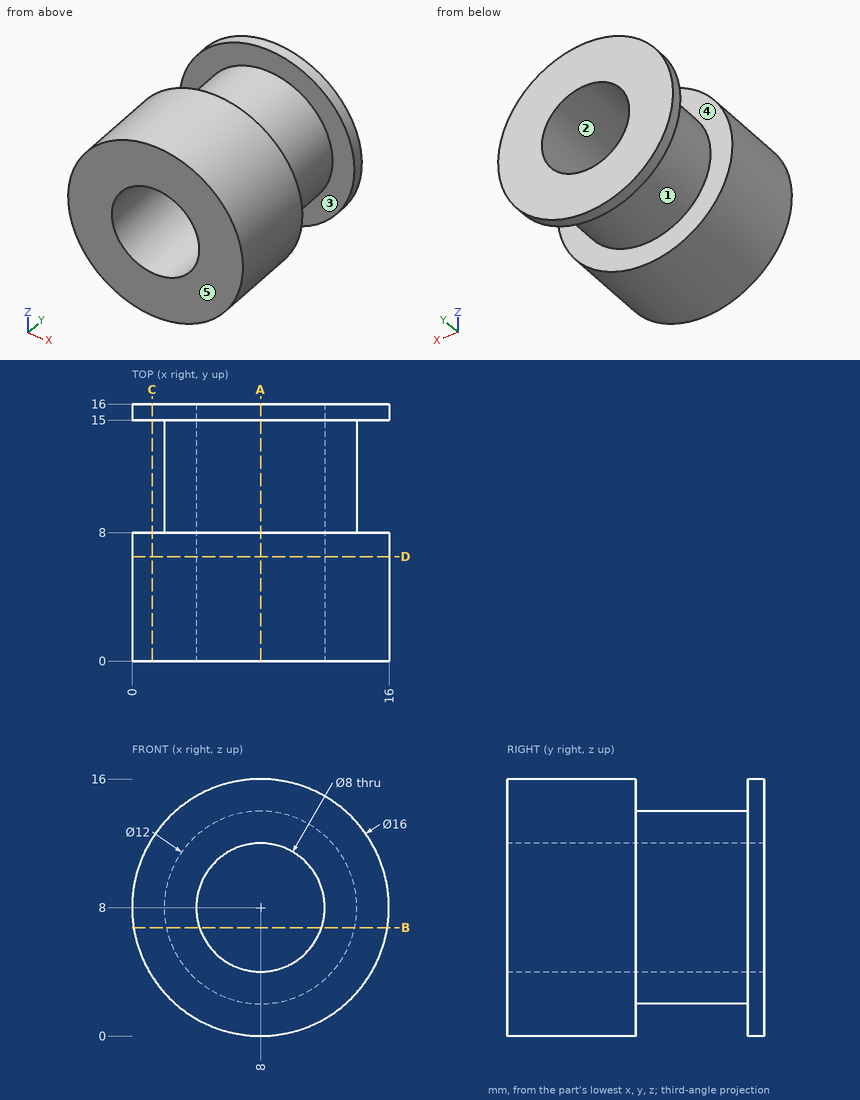
Input: dimensioned drawing with shaded views. Units: mm. Origin: part minimum x, y, z. A direction names the side the tool comes from. Give positions to 0.01 mm unless a question says otherwise; leave off trailing zeros. Write each loop counter-clockwise with the first axis right and the second up, starting at its lowest first coordinate (ties: lowest second). Pieces come first, ordered by that corner, then holes. Notation, with made-up numbers: M -34,40.25 L -25,40.25 A13 ccw -25,48.25 Z; hole C 43.25,-39.5 d10. An arc over 180 degrees is marked long. Write item = value, one per line. Start each with the question number.
1) Material intervals for line 1 along Y through (x, z) = (11, 14.5); line 2 along X through (y, z) = (8.75, 8); line 3 along X through (y, z) = (7.5, 8), sorted ascending. Write a range as [from, to].
2) Cut plane B-B on z = 6.75. Return the cut outline in (x, y), then the cut area to 3 significant figures.
3) Reachability of the marked faces 4 and 5 from +Z, -Z, +X, -X, +Y, -Y: full face, straight path, thin tool, end or side. Return the list, or none.
4) Cut plane A-A on x = 8. Return the cut outline in (y, z).
5) Cut plane C-C on x = 1.25. Return the cut outline in (y, z), then the cut area to 3 significant figures.
6) First-contact query: pin 1 Ø1 at (y, z) = (3, 4) entering from -X; pin 2 Ø1.5 at (y, z) = (9.5, 4.5) entering from -X; pin 3 Ø2 at (y, z) = (3, 3) entering from -X. Flat tips, straight axial feed; report the tip coordinate or a pass-through.
7) Cut plane D-D on y = 6.5. Return the cut outline in (x, z), then the cut area to 3 significant figures.
8) Draft query along Z for the marked faces 1, 2 and 3. Return one class per face: +Z half, -Z half, draft (parallel to the pull), parting line (faces both ways), or undercut.
Solved:
q1.line_1 = [0, 8], [15, 16]
q1.line_2 = [2, 4], [12, 14]
q1.line_3 = [0, 4], [12, 16]
q2.outline = M 0.1,0 L 4.2,0 L 4.2,16 L 0.1,16 L 0.1,15 L 2.13,15 L 2.13,8 L 0.1,8 Z; M 11.8,0 L 15.9,0 L 15.9,8 L 13.87,8 L 13.87,15 L 15.9,15 L 15.9,16 L 11.8,16 Z
q2.area = 103 mm2
q3.face_4 = none
q3.face_5 = +Z, -Z, +X, -X, -Y
q4.outline = M 0,0 L 8,0 L 8,2 L 15,2 L 15,0 L 16,0 L 16,4 L 0,4 Z; M 0,12 L 16,12 L 16,16 L 15,16 L 15,14 L 8,14 L 8,16 L 0,16 Z
q5.outline = M 0,3.71 L 8,3.71 L 8,12.29 L 0,12.29 Z; M 15,3.71 L 16,3.71 L 16,12.29 L 15,12.29 Z
q5.area = 77.3 mm2
q6.pin_1 = 0.81
q6.pin_2 = 2.67
q6.pin_3 = 1.07
q7.outline = C 8,8 d16; hole C 8,8 d8
q7.area = 151 mm2
q8.face_1 = parting line
q8.face_2 = undercut
q8.face_3 = draft
